Can you work these out from the model? Positions are in its coordinate system, mm. Round coordinates to 2 decimals unless told otherwise and drop trailing zeros. Loops run counter-clockwise (first coordinate to the right, second up) from the corner with the lowest first, then second, coordinate; pieces in that order, holes last. Notation, with made-up numbers: (8, 83) -> (37, 83) arc R14 cw to (37, 93) -> close; hole circle Ø7 at (-4, 58.25). An arc over 180 degrees is marked (long way). Write item = value, one per line.
from build123d import *

# Parameters (mm, degrees)
SKETCH1_W           = 177.8
SKETCH1_H           = 6.35
BOSS_EXTRUDE1_DEPTH = 3.175
FILLET1_R           = 2.54
CUT_EXTRUDE1_REACH  = 91.013
SKETCH2_R           = 2.032


with BuildPart() as part:
    # Sketch1 → Boss-Extrude1 (new body)
    with BuildSketch(Plane(origin=(0, 0, 0), x_dir=(1, 0, 0), z_dir=(0, 1, 0))):
        Rectangle(SKETCH1_W, SKETCH1_H)
    extrude(amount=BOSS_EXTRUDE1_DEPTH)

    # Fillet1
    fillet1_edges = [part.edges().sort_by_distance(p)[0] for p in [
        (-88.9, 1.5875, 3.175),
        (-88.9, 1.5875, -3.175),
        (88.9, 1.5875, -3.175),
        (88.9, 1.5875, 3.175),
    ]]
    fillet(fillet1_edges, radius=FILLET1_R)

    # Sketch2 → Cut-Extrude1 (cut, up to next)
    with BuildSketch(Plane(origin=(0, 3.175, 0), x_dir=(1, 0, 0), z_dir=(0, 1, 0)), mode=Mode.PRIVATE) as cut_extrude1_sk1:
        with Locations(Location((-76.2, 0, 0), (0, 0, 270))):
            Circle(SKETCH2_R)
    cut_extrude1_tool1 = extrude(cut_extrude1_sk1.sketch, amount=-CUT_EXTRUDE1_REACH, mode=Mode.PRIVATE) & part.part
    # Sketch2 → Cut-Extrude1 (cut, up to next)
    with BuildSketch(Plane(origin=(0, 3.175, 0), x_dir=(1, 0, 0), z_dir=(0, 1, 0)), mode=Mode.PRIVATE) as cut_extrude1_sk2:
        with Locations(Location((0, 0, 0), (0, 0, 270))):
            Circle(SKETCH2_R)
    cut_extrude1_tool2 = extrude(cut_extrude1_sk2.sketch, amount=-CUT_EXTRUDE1_REACH, mode=Mode.PRIVATE) & part.part
    # Sketch2 → Cut-Extrude1 (cut, up to next)
    with BuildSketch(Plane(origin=(0, 3.175, 0), x_dir=(1, 0, 0), z_dir=(0, 1, 0)), mode=Mode.PRIVATE) as cut_extrude1_sk3:
        with Locations(Location((-38.1, 0, 0), (0, 0, 270))):
            Circle(SKETCH2_R)
    cut_extrude1_tool3 = extrude(cut_extrude1_sk3.sketch, amount=-CUT_EXTRUDE1_REACH, mode=Mode.PRIVATE) & part.part
    # Sketch2 → Cut-Extrude1 (cut, up to next)
    with BuildSketch(Plane(origin=(0, 3.175, 0), x_dir=(1, 0, 0), z_dir=(0, 1, 0)), mode=Mode.PRIVATE) as cut_extrude1_sk4:
        with Locations(Location((83.82, 0, 0), (0, 0, 270))):
            Circle(SKETCH2_R)
    cut_extrude1_tool4 = extrude(cut_extrude1_sk4.sketch, amount=-CUT_EXTRUDE1_REACH, mode=Mode.PRIVATE) & part.part
    # Sketch2 → Cut-Extrude1 (cut, up to next)
    with BuildSketch(Plane(origin=(0, 3.175, 0), x_dir=(1, 0, 0), z_dir=(0, 1, 0)), mode=Mode.PRIVATE) as cut_extrude1_sk5:
        with Locations(Location((54.61, 0, 0), (0, 0, 270))):
            Circle(SKETCH2_R)
    cut_extrude1_tool5 = extrude(cut_extrude1_sk5.sketch, amount=-CUT_EXTRUDE1_REACH, mode=Mode.PRIVATE) & part.part
    # Sketch2 → Cut-Extrude1 (cut, up to next)
    with BuildSketch(Plane(origin=(0, 3.175, 0), x_dir=(1, 0, 0), z_dir=(0, 1, 0)), mode=Mode.PRIVATE) as cut_extrude1_sk6:
        with Locations(Location((34.29, 0, 0), (0, 0, 270))):
            Circle(SKETCH2_R)
    cut_extrude1_tool6 = extrude(cut_extrude1_sk6.sketch, amount=-CUT_EXTRUDE1_REACH, mode=Mode.PRIVATE) & part.part
    add(cut_extrude1_tool1.solids().sort_by_distance((-76.2, 3.175, 0))[0], mode=Mode.SUBTRACT)
    add(cut_extrude1_tool2.solids().sort_by_distance((0, 3.175, 0))[0], mode=Mode.SUBTRACT)
    add(cut_extrude1_tool3.solids().sort_by_distance((-38.1, 3.175, 0))[0], mode=Mode.SUBTRACT)
    add(cut_extrude1_tool4.solids().sort_by_distance((83.82, 3.175, 0))[0], mode=Mode.SUBTRACT)
    add(cut_extrude1_tool5.solids().sort_by_distance((54.61, 3.175, 0))[0], mode=Mode.SUBTRACT)
    add(cut_extrude1_tool6.solids().sort_by_distance((34.29, 3.175, 0))[0], mode=Mode.SUBTRACT)


solid = part.part
1. We'd pull the mould along Z, two halves only. Please class faces 1 (the flat face through (-1, 3.175, -2)), 2 (the cylindrical face through (52.81, 1.61, 0.94)), 3 (the flat face through (-1, 2, -3.175)): released by +Z, released by -Z, zero draft, split by the parting line, or undercut.
Entries:
face_1 = zero draft
face_2 = undercut
face_3 = released by -Z
2. I need wall thicknesses on line 1 (Z direction, x = -1.5, y = 1.15) (3 decimals); line 2 (X direction, y = 2.35, z = 2.75). Which ranges of each line are inside material? Lowest first, please. Write a range as [from, to].
Entries:
line_1 = [-3.175, -1.371], [1.371, 3.175]
line_2 = [-87.77, 87.77]
3. Suppose I cut it at A-A, the plane y = 1.6. List the corners of the cut face in (x, z) for me (3 decimals).
Entries:
outline = (-88.9, -0.635) arc R2.54 ccw to (-86.36, -3.175) -> (86.36, -3.175) arc R2.54 ccw to (88.9, -0.635) -> (88.9, 0.635) arc R2.54 ccw to (86.36, 3.175) -> (-86.36, 3.175) arc R2.54 ccw to (-88.9, 0.635) -> close; hole circle Ø4.064 at (-76.2, 0); hole circle Ø4.064 at (-38.1, 0); hole circle Ø4.064 at (0, 0); hole circle Ø4.064 at (34.29, 0); hole circle Ø4.064 at (54.61, 0); hole circle Ø4.064 at (83.82, 0)
4. Suppose I cut it at B-B, the plane x = -76.2. List the corners of the cut face in (y, z) for me (3 decimals).
Entries:
outline = (0, -3.175) -> (3.175, -3.175) -> (3.175, -2.032) -> (0, -2.032) -> close; (0, 2.032) -> (3.175, 2.032) -> (3.175, 3.175) -> (0, 3.175) -> close
